Check sheet for the drawn part. Datum: minimum x, y, z corner. Units: mm. A direction names the side the tool comes from. Coordinates: 2 decimals unless noted, no trailing zeros. Order: outer loops, then holes, each group sorted by start corner. A loop starts at its lowest first (then second) coordinate and runs counter-clockwise, first axis right, second up.
1. Cross-section at D-D (y = 17). Enter the section's corners in (x, z), then the cut area to 3 significant figures.
2. Cross-section at B-B (x = 2.5). Enter the section's corners in (y, z).
3. Cross-section at A-A (z = 2.5). Enter the section's corners in (x, y), then the cut area to 3 significant figures.
4. Gauge pin test, flat ends, axial feed: pin 1 Ø2 at (x, y) = (1.5, 13.5) entering from +Z; pin 2 Ø3 at (y, z) = (7.5, 4.5) entering from +X. Record the tip position at first contact, or that the pin passes through.
5. Cross-section at C-C (y = 8.25). Enter the section's corners in (x, z), then the cut area to 3 significant figures.
6. Set-up check for the marked faces 1, 2 and 3: record each of +Z, -Z, +X, -X, +Y, -Y from which the full face is reachable in a straight line by a thin tool's end or side.
7. Thickness scan on line 1 (Y direction, x = 0.4, z = 3.6); line 2 (Z direction, x = 2.1, y = 9); line 3 (X direction, y = 16.25, z = 2.2). Record the ranges inside material, lowest first.
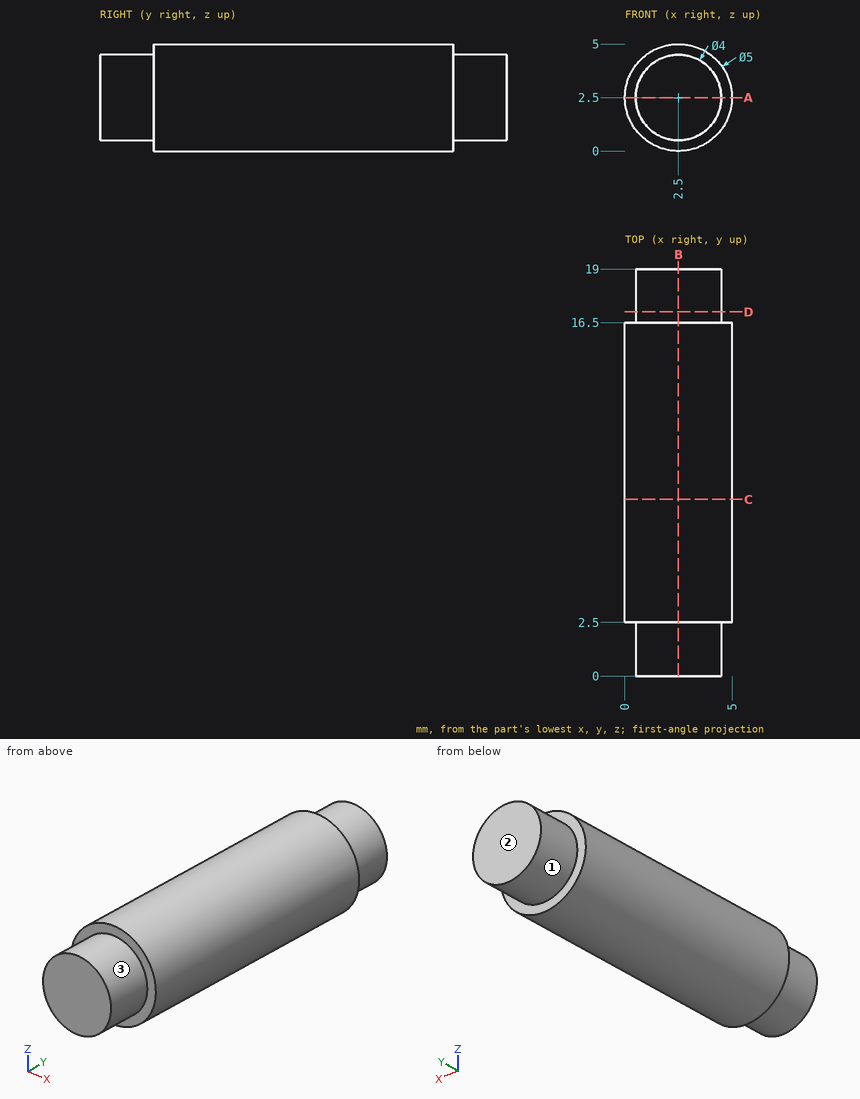
Data:
1. outline: circle Ø4 at (2.5, 2.5)
1. area: 12.6 mm2
2. outline: (0, 0.5) - (2.5, 0.5) - (2.5, 0) - (16.5, 0) - (16.5, 0.5) - (19, 0.5) - (19, 4.5) - (16.5, 4.5) - (16.5, 5) - (2.5, 5) - (2.5, 4.5) - (0, 4.5) - close
3. outline: (0, 2.5) - (0.5, 2.5) - (0.5, 0) - (4.5, 0) - (4.5, 2.5) - (5, 2.5) - (5, 16.5) - (4.5, 16.5) - (4.5, 19) - (0.5, 19) - (0.5, 16.5) - (0, 16.5) - close
3. area: 90.0 mm2
4. pin 1: stops at z = 5
4. pin 2: stops at x = 4.95
5. outline: circle Ø5 at (2.5, 2.5)
5. area: 19.6 mm2
6. face 1: +Y
6. face 2: +Z, -Z, +X, -X, +Y
6. face 3: -Y
7. line 1: y = 2.5 to 16.5
7. line 2: z = 0.03 to 4.97
7. line 3: x = 0.02 to 4.98
